Could you check a few things on this model? Use its own coordinates, in mm. Face numbers are marked on the shaded views. Give positions to 0.01 mm unless a question says otherwise; leave off trailing zeros. Loops run counter-clockwise (first coordinate to the right, second up) from the corner with the lowest first, then second, coordinate; pieces in that order, holes last.
1. Imagine slicing it at D-D (x = 45). List the corners of the cut face in (y, z) for me, plus the area to 3 significant figures.
2. For P1, Ø1, axis at x = 36, y = 32, coming from the +Z side; P2, Ø4, axis at y = 36, z = -8, coming from the +X side; P3, Ø1.5, axis at y = 28.5, z = -5.5, coming from the -X side, each with a flat end and sliding along its axis, tell me the tip position at first contact or that it passes through.
3. Thinking about a two-plate mould opening in Z: for the marked faces 1, 2 and 3, which applies, +Z half, -Z half, draft (parallel to the pull), parting line (faces both ways), or undercut?
4. Imagine slicing it at A-A (x = 67). List the corners of the cut face in (y, z) for me.
5. Imagine slicing it at C-C (y = 32.5). List the corners of the cut face in (x, z) for me, plus the area to 3 significant figures.
6. I need wall thicknesses on line 1 along Y through (x, z) = (46, -3.5); line 2 along X through (y, z) = (39, -6.5); line 3 along Z through (x, y) = (39, 10). Which ranges of each line are inside material? Lowest first, please.
7. Imagine slicing it at B-B (z = -15.75). List the corners of the cut face in (x, y) for me (3 decimals).
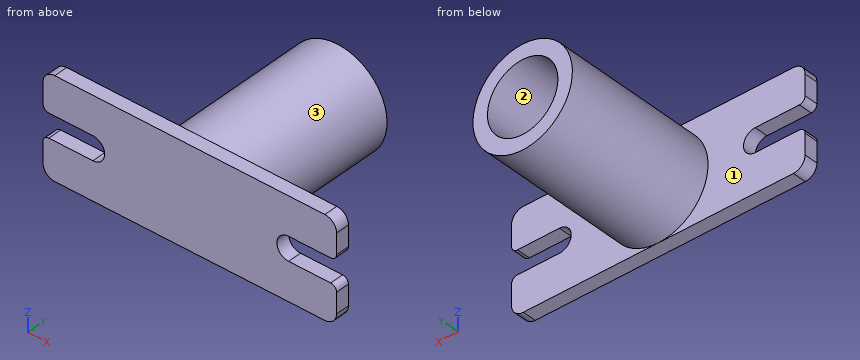
```python
from build123d import *

# Parameters (mm, degrees)
BOSS_EXTRUDE2_DEPTH = 3.5
SKETCH4_R           = 12.7
BOSS_EXTRUDE3_DEPTH = 15
SKETCH5_R           = 12.7
SKETCH5_R_2         = 9
BOSS_EXTRUDE4_DEPTH = 25


with BuildPart() as part:
    # Sketch1 → Boss-Extrude2 (new body)
    with BuildSketch(Plane(origin=(0, 0, 0), x_dir=(1, 0, 0), z_dir=(0, 1, 0))):
        with BuildLine():
            Line((64.453053112, 11.100827963), (75.203053112, 11.100827963))
            ThreePointArc((75.203053112, 11.100827963), (76.263713284, 11.540167791), (76.703053112, 12.600827963))
            Line((76.703053112, 12.600827963), (76.703053112, 17.800827963))
            ThreePointArc((76.703053112, 17.800827963), (75.824373455, 19.922148306), (73.703053112, 20.800827963))
            Line((73.703053112, 20.800827963), (4.703053112, 20.800827963))
            ThreePointArc((4.703053112, 20.800827963), (2.581732768, 19.922148306), (1.703053112, 17.800827963))
            Line((1.703053112, 17.800827963), (1.703053112, 12.600827963))
            ThreePointArc((1.703053112, 12.600827963), (2.14239294, 11.540167791), (3.203053112, 11.100827963))
            Line((3.203053112, 11.100827963), (14.453053112, 11.100827963))
            ThreePointArc((14.453053112, 11.100827963), (17.453053112, 8.100827963), (14.453053112, 5.100827963))
            Line((14.453053112, 5.100827963), (3.203053112, 5.100827963))
            ThreePointArc((3.203053112, 5.100827963), (2.14239294, 4.661488134), (1.703053112, 3.600827963))
            Line((1.703053112, 3.600827963), (1.703053112, -1.599172037))
            ThreePointArc((1.703053112, -1.599172037), (2.581732768, -3.720492381), (4.703053112, -4.599172037))
            Line((4.703053112, -4.599172037), (73.703053112, -4.599172037))
            ThreePointArc((73.703053112, -4.599172037), (75.824373455, -3.720492381), (76.703053112, -1.599172037))
            Line((76.703053112, -1.599172037), (76.703053112, 3.600827963))
            ThreePointArc((76.703053112, 3.600827963), (76.263713284, 4.661488134), (75.203053112, 5.100827963))
            Line((75.203053112, 5.100827963), (64.453053112, 5.100827963))
            ThreePointArc((64.453053112, 5.100827963), (61.453053112, 8.100827963), (64.453053112, 11.100827963))
        make_face()
    extrude(amount=BOSS_EXTRUDE2_DEPTH)

    # Sketch4 → Boss-Extrude3 (add)
    with BuildSketch(Plane(origin=(0, 3.5, 0), x_dir=(1, 0, 0), z_dir=(0, 1, 0))):
        with Locations(Location((39.203053112, 8.100827963, 0), (0, 0, 270))):
            Circle(SKETCH4_R)
    extrude(amount=BOSS_EXTRUDE3_DEPTH)

    # Sketch5 → Boss-Extrude4 (add)
    with BuildSketch(Plane(origin=(0, 18.5, 0), x_dir=(1, 0, 0), z_dir=(0, 1, 0))):
        with Locations(Location((39.203053112, 8.100827963, 0), (0, 0, 270))):
            Circle(SKETCH5_R)
        with Locations(Location((39.203053112, 8.100827963, 0), (0, 0, 270))):
            Circle(SKETCH5_R_2, mode=Mode.SUBTRACT)
    extrude(amount=BOSS_EXTRUDE4_DEPTH)


solid = part.part
```
Derived:
1. outline: (0, -20.8) - (3.5, -20.8) - (3.5, -19.4) - (43.5, -19.4) - (43.5, -14.99) - (18.5, -14.99) - (18.5, -1.22) - (43.5, -1.22) - (43.5, 3.2) - (3.5, 3.2) - (3.5, 4.6) - (0, 4.6) - close
1. area: 649 mm2
2. P1: stops at z = 4.31
2. P2: stops at x = 51.9
2. P3: stops at x = 26.64
3. face 1: draft
3. face 2: undercut
3. face 3: parting line
4. outline: (0, -20.8) - (3.5, -20.8) - (3.5, -11.1) - (0, -11.1) - close; (0, -5.1) - (3.5, -5.1) - (3.5, 4.6) - (0, 4.6) - close
5. outline: circle Ø25.4 at (39.2, -8.1); hole circle Ø18 at (39.2, -8.1)
5. area: 252 mm2
6. line 1: y = 0 to 18.5
6. line 2: x = 26.6 to 30.35, 48.06 to 51.8
6. line 3: z = -20.8 to 4.6
7. outline: (1.703, 0) - (76.703, 0) - (76.703, 3.5) - (49.341, 3.5) - (49.341, 43.5) - (43.945, 43.5) - (43.945, 18.5) - (34.461, 18.5) - (34.461, 43.5) - (29.065, 43.5) - (29.065, 3.5) - (1.703, 3.5) - close
